Autodesk Inventor part; units mm, degrees
ref_plane "YZ Plane" through (0, 0, 0) normal (1, 0, 0) x (0, 1, 0)
ref_plane "XZ Plane" through (0, 0, 0) normal (0, 1, 0) x (-1, 0, 0)
ref_plane "XY Plane" through (0, 0, 0) normal (0, 0, 1) x (1, 0, 0)
sketch "Esquisse1" plane through (0, 0, 0) normal (0, 0, 1) x (1, 0, 0)
  circle A0 centre (0, 0) radius 2
  line L0 (0, 0) -> (46.5696, 0) construction
  line L1 (0, 0) -> (27.5772, 27.5772) construction
  circle A1 centre (27.5772, 27.5772) radius 2
  line L2 (27.5772, 27.5772) -> (55.1548, 4.4368) construction
  line L3 (27.5772, 27.5772) -> (45.4581, 27.5772) construction
  line L4 (0, 0) -> (0, -8) construction
  line L5 (0, 0) -> (-5.6569, 5.6569) construction
  line L6 (27.5772, 27.5772) -> (27.5772, 35.5772) construction
  line L7 (27.5772, 27.5772) -> (36.2548, 37.9188) construction
  line L8 (36.2548, 37.9188) -> (41.2341, 33.7406) construction
  line L9 (41.2341, 33.7406) -> (47.3624, 28.5983) construction
  line L10 (47.3624, 28.5983) -> (53.4908, 23.456) construction
  line L11 (53.4908, 23.456) -> (59.6192, 18.3137) construction
  line L12 (55.1548, 4.4368) -> (60.2971, 10.5652) construction
  circle A2 centre (41.2341, 33.7406) radius 1 construction
  circle A3 centre (47.3624, 28.5983) radius 1
  circle A4 centre (53.4908, 23.456) radius 1
  circle A5 centre (59.6192, 18.3137) radius 1
  circle A6 centre (60.2971, 10.5652) radius 1
  line L13 (59.6192, 18.3137) -> (67.6192, 18.3137) construction
  line L14 (67.6192, 35.5772) -> (67.6192, -8)
  line L15 (67.6192, -8) -> (-17.1163, -8)
  line L16 (-17.1163, -8) -> (19.4493, 35.5772)
  line L17 (19.4493, 35.5772) -> (67.6192, 35.5772)
  circle A7 centre (23.8788, 13.0574) radius 1 construction
  circle A8 centre (30.0072, 7.9151) radius 1
  circle A9 centre (36.1355, 2.7728) radius 1
  circle A10 centre (42.2639, -2.3695) radius 1
  circle A11 centre (50.0125, -1.6915) radius 1
  line L18 (0, 0) -> (25, 0) construction
  circle A12 centre (25, 0) radius 2
  dimension "d0" = 4
  dimension "d1" = 39
  dimension "d2" = 45
  dimension "d3" = 36
  dimension "d4" = 40
  dimension "d5" = 8
  dimension "d6" = 8
  dimension "d7" = 8
  dimension "d8" = 13.5
  dimension "d9" = 6.5
  dimension "d10" = 8
  dimension "d11" = 8
  dimension "d12" = 8
  dimension "d13" = 8
  dimension "d14" = 2
  dimension "d15" = 8
  dimension "d16" = 25
extrude "Extrusion1" add sketch "Esquisse1" along normal blind 12
sketch "Esquisse4" plane through (0, 0, 12) normal (0, 0, 1) x (1, 0, 0)
  circle A0 centre (27.5772, 27.5772) radius 2
  circle A1 centre (0, 0) radius 2
  line L0 (67.6192, 35.5772) -> (19.4493, 35.5772)
  line L1 (19.4493, 35.5772) -> (-17.1163, -8)
  circle A2 centre (27.5772, 27.5772) radius 12 construction
  line L2 (39.5772, 35.5772) -> (39.5772, 27.5772)
  line L3 (30.5997, 15.964) -> (-4.7219, 6.771)
  arc A3 (30.5997, 15.964) -> (39.5772, 27.5772) centre (27.5772, 27.5772) ccw
  line L4 (-17.1163, -8) -> (67.6192, -8)
  line L5 (0, 0) -> (0, 8) construction
  dimension "d42" = 24
  dimension "d51" = 8
extrude "Extrusion4" cut sketch "Esquisse4" against normal blind 7 contours L2 A3 L3 L1 L0
sketch "Esquisse5" plane through (0, 0, 12) normal (0, 0, 1) x (1, 0, 0)
  line L0 (67.6192, -8) -> (67.6192, 35.5772)
  circle A0 centre (0, 0) radius 2
  circle A1 centre (25, 0) radius 2
  line L1 (28.5, -2.0207) -> (25, -4.0415)
  line L2 (25, -4.0415) -> (21.5, -2.0207)
  line L3 (21.5, -2.0207) -> (21.5, 2.0207)
  line L4 (21.5, 2.0207) -> (25, 4.0415)
  line L5 (25, 4.0415) -> (28.5, 2.0207)
  line L6 (28.5, 2.0207) -> (28.5, -2.0207)
  line L7 (3.5, -2.0207) -> (0, -4.0415)
  line L8 (0, -4.0415) -> (-3.5, -2.0207)
  line L9 (-3.5, -2.0207) -> (-3.5, 2.0207)
  line L10 (-3.5, 2.0207) -> (0, 4.0415)
  line L11 (0, 4.0415) -> (3.5, 2.0207)
  line L12 (3.5, 2.0207) -> (3.5, -2.0207)
  line L13 (21.5, 2.0207) -> (28.5, 2.0207) construction
  dimension "d46" = 7
extrude "Extrusion5" cut sketch "Esquisse5" against normal blind 3
sketch "Esquisse6" plane through (0, 0, 5) normal (0, 0, 1) x (1, 0, 0)
  circle A0 centre (27.5772, 27.5772) radius 2
  arc A1 (30.5997, 15.964) -> (39.5772, 27.5772) centre (27.5772, 27.5772) ccw
  line L0 (31.0772, 29.5979) -> (31.0772, 25.5564)
  line L1 (31.0772, 25.5564) -> (27.5772, 23.5357)
  line L2 (27.5772, 23.5357) -> (24.0772, 25.5564)
  line L3 (24.0772, 25.5564) -> (24.0772, 29.5979)
  line L4 (24.0772, 29.5979) -> (27.5772, 31.6186)
  line L5 (27.5772, 31.6186) -> (31.0772, 29.5979)
  line L6 (67.6192, -8) -> (67.6192, 35.5772)
  line L7 (0, 4.0415) -> (3.5, 2.0207)
  point P0 (0, 0)
extrude "Extrusion6" cut sketch "Esquisse6" against normal blind 3
fillet "Congé10" radius 8 1 edges at (-17.1163, -8, 6)
chamfer "Chanfrein3" distance 15 angle 45 1 edges at (67.6192, -8, 6)
chamfer "Chanfrein4" distance 15 angle 45 1 edges at (67.6192, 35.5772, 6)
fillet "Congé11" radius 10 1 edges at (52.6192, -8, 6)
fillet "Congé12" radius 10 1 edges at (67.6192, 7, 6)
fillet "Congé13" radius 10 1 edges at (67.6192, 20.5772, 6)
fillet "Congé14" radius 10 1 edges at (52.6192, 35.5772, 6)
fillet "Congé15" radius 10 1 edges at (19.4493, 35.5772, 2.5)
fillet "Congé16" radius 8 1 edges at (39.5772, 35.5772, 8.5)
properties part number "joint1right+ax12imprint_v3"
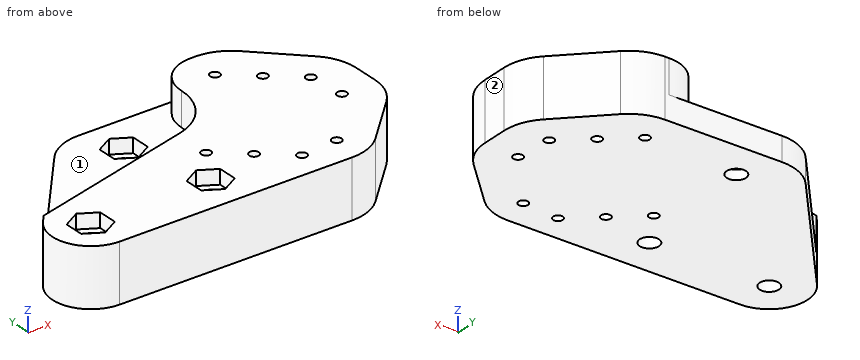
Work out the finished part from the listing and answer in its coordinate system (mm). Face numbers are marked on the shaded views. A direction names the side the tool comes from. Coordinates: 2 decimals unless noted, no trailing zeros. Write each loop counter-clockwise with the first axis right and the second up, starting at its lowest first coordinate (ties: lowest second). Pieces come first, ordered by that corner, then holes.
1. The part is cut by section A-A, the plane z = 3. State how many separate pieces and enclosed holes the cut face has, and give its area (3 significant figures).
Results list:
separate pieces: 1
enclosed holes: 11
area: 2,500 mm2
2. Flat-ended cylindrical pins translate along their axes: pin 1 (1.5 mm diameter, centred on y = 0, z = 10, fed in from +X); pin 2 (1.5 mm diameter, centred on x = 2, z = 7.5, fed in from +Y); pin 3 (0.9 mm diameter, centred on y = 0, z = 10.5, fed in from +X). Find the tip coordinate at first contact, or state that the pin passes through.
Results list:
pin 1: stops at x = 61.37
pin 2: stops at y = 8.72
pin 3: stops at x = 61.07
3. For the marked faces 1 and 2, determine the directions among +Z, -Z, +X, -X, +Y, -Y from which every point of the face is accessible in a straight line to the end or side of a thin tool.
Results list:
face 1: +Z, -X, +Y
face 2: +Z, -Z, +X, +Y, -Y
4. The part is cut by section C-C, the plane x = 56.5. Write down the section's boundary in (y, z).
Results list:
outline: (-4.12, 0) - (31.7, 0) - (31.7, 12) - (-4.12, 12) - close
5. Consider line 1 along Y through (x, z) = (25, 3); line 2 along X through (y, z) = (24, 3); line 3 along Y through (x, z) = (53, 7.75). Determine where each line is inside the solid, lowest interval first.
Results list:
line 1: y = -8 to -2, 2 to 25.02, 30.13 to 35.58
line 2: x = 9.73 to 26.77, 28.38 to 52.65, 54.33 to 64.2
line 3: y = -6.92 to 22.58, 24.33 to 34.5
